from build123d import *

# Parameters (mm, degrees)
F1_DEPTH = 265.1125
F2_R     = 5.08
F3_R     = 7.14375
F4_DEPTH = 25.4


with BuildPart() as f1:
    # F0 (on Front) → F1 (new body, symmetric)
    with BuildSketch(Plane.XZ):
        Polygon((0, 76.2), (0, 0), (76.2, 0), (76.2, 9.525), (9.525, 9.525), (9.525, 76.2), align=None)
    extrude(amount=F1_DEPTH, both=True)

    # F2
    f2_edges = [f1.edges().sort_by_distance(p)[0] for p in [
        (9.525, 0, 76.2),
        (9.525, 0, 9.525),
        (76.2, 0, 9.525),
    ]]
    fillet(f2_edges, radius=F2_R)

    # F3 (on face) → F4 (cut)
    with BuildSketch(Plane(origin=(0, 0, 0), x_dir=(0, -1, 0), z_dir=(-1, 0, 0))):
        with Locations((-98.425, 38.1)):
            Circle(F3_R)
        with Locations((98.425, 38.1)):
            Circle(F3_R)
    extrude(amount=-F4_DEPTH, mode=Mode.SUBTRACT)


solid = f1.part
Verification items for the finished model (mm, model axes). A direction names the side the tool comes from. Give positions to 0.01 mm unless a question says otherwise; leave off trailing zeros. Loops run counter-clockwise (first coordinate to the right, second up) from the corner with the lowest first, then second, coordinate; pieces in that order, holes last. Notation, with made-up numbers: (8.25, -30.75) - (36.25, -30.75) arc R15 ccw to (36.25, -9.75) - close; hole circle Ø8 at (49.5, -2). An arc over 180 degrees is marked (long way). Write item = value, one per line. Start each with the question number.
Q1. Cross-section at B-B, the plane y = 35. Enter the section's corners in (x, z) (3 decimals).
Q2. Cross-section at C-C, the plane x = 30. Enter the section's corners in (y, z) (1 decimal).
Q3. Cross-section at A-A, the plane z = 38.1. Enter the section's corners in (x, y) (1 decimal).
Q4. Tool access check on faces 5 (the face through (38, -4, 0)), 6 (the face through (9.525, -4, 42)). Record the directions out of +Z, -Z, +X, -X, +Y, -Y that give a thin tool (end or side, any length) a straight path to the whole face; none if there is none.
Q5. Depth check by flat-ended pin: P1, Ø3, axis at y = 25.5, z = 33.5, coming from the +X side (3 decimals); P2, Ø4, axis at x = 26.5, y = 51, coming from the +Z side (3 decimals). Enter the tip coordinate at first touch or a pass-through.
Q6. Mould release check, pull along Y, two halves, no side actions. Record for faces 1 (the face through (24, -265.112, 7)), 2 (the face through (4.7, 94.58, 44.12)), 3 (the face through (24, 265.112, 7)), 4 (the face through (43, -4, 9.525)): released by +Y, released by -Y, zero draft, split by the parting line, or undercut.
Q7. Thickness scan on line 1 (Y direction, x = 2, z = 38); line 2 (X direction, y = 182, z = 49) (3 decimals). Record the ranges inside material, lowest first.
Answer key:
q1.outline = (0, 0) - (76.2, 0) - (76.2, 4.445) arc R5.08 ccw to (71.12, 9.525) - (14.605, 9.525) arc R5.08 cw to (9.525, 14.605) - (9.525, 71.12) arc R5.08 ccw to (4.445, 76.2) - (0, 76.2) - close
q2.outline = (-265.1, 0) - (265.1, 0) - (265.1, 9.5) - (-265.1, 9.5) - close
q3.outline = (0, -265.1) - (9.5, -265.1) - (9.5, -105.6) - (0, -105.6) - close; (0, -91.3) - (9.5, -91.3) - (9.5, 91.3) - (0, 91.3) - close; (0, 105.6) - (9.5, 105.6) - (9.5, 265.1) - (0, 265.1) - close
q4.face_5 = -Z, +X, -X, +Y, -Y
q4.face_6 = +Z, +X, +Y, -Y
q5.P1 = 9.525
q5.P2 = 9.525
q6.face_1 = released by -Y
q6.face_2 = undercut
q6.face_3 = released by +Y
q6.face_4 = zero draft
q7.line_1 = -265.11 to -105.57, -91.28 to 91.28, 105.57 to 265.11
q7.line_2 = 0 to 9.525
